from build123d import *

# Parameters (mm, degrees)
F0_R     = 5.35
F1_DEPTH = 1.5
F2_R     = 4.73
F3_DEPTH = 6.16
F4_R     = 1.13
F5_DEPTH = 2.18
F6_R     = 2.97
F7_DEPTH = 13.4
F8_SIZE  = 0.25


with BuildPart() as f1:
    # F0 (on Front) → F1 (new body)
    with BuildSketch(Plane.XZ):
        Circle(F0_R)
    extrude(amount=F1_DEPTH)

    # F2 (on face) → F3 (join)
    with BuildSketch(Plane.XZ.offset(1.5)):
        Circle(F2_R)
    extrude(amount=F3_DEPTH)

    # F4 (on face) → F5 (join)
    with BuildSketch(Plane.XZ.offset(7.66)):
        Circle(F4_R)
    extrude(amount=F5_DEPTH)

    # F6 (on face) → F7 (join)
    with BuildSketch(Plane(origin=(0, 0, 0), x_dir=(-1, 0, 0), z_dir=(0, 1, 0))):
        Circle(F6_R)
    extrude(amount=F7_DEPTH)

    # F8
    f8_edges = [f1.edges().sort_by_distance(p)[0] for p in [
        (-4.73, -7.66, 0),
        (2.97, 13.4, 0),
    ]]
    chamfer(f8_edges, length=F8_SIZE)


solid = f1.part
Work out the finished part from the listing and answer in its coordinate system (mm). A direction names the side the tool comes from. Give positions to 0.01 mm unless a question says otherwise; leave off trailing zeros. Order: outer loops, then holes, each group sorted by start corner. A loop starts at its lowest first (then second) coordinate and runs counter-clockwise, first axis right, second up. Notation, with made-up numbers: M -16.5,75.25 L 30.5,75.25 A24 ccw 30.5,96.25 Z; hole C 15,-38.75 d4. An arc over 180 degrees is marked long. Return JSON: item names as keys, results as strings.
Q1. Which of the six approach directions +Z, -Z, +X, -X, +Y, -Y give full straight-line access (tool end or side, diameter ignored) to faces 1 (the face through (2.3, 0, -2.3)), 2 (the face through (1, -7.66, -1)), 3 (the face through (0, -9.84, 0))?
Answer below:
{"face 1": "+Y", "face 2": "-Y", "face 3": "+Z, -Z, +X, -X, -Y"}
Q2. Find the intervals of material crossed by line 1 along Y through (x, z) = (4, -1.5); line 2 along Y through (x, z) = (0.5, 1.5); line 3 along X through (y, z) = (4.5, -0.75), in increasing order. Write a range as [from, to].
Answer below:
{"line 1": "y = [-7.66, 0]", "line 2": "y = [-7.66, 13.4]", "line 3": "x = [-2.87, 2.87]"}
Q3. Find section C-C, the plane y = -1.25. Write down the section's boundary in (x, z), and give its area (3 significant figures).
Answer below:
{"outline": "C 0,0 d10.7", "area": "89.9 mm^2"}
Q4. Each of these flat-tipped pins is pushed along its axis until it touches: pin 1 (3 mm diameter, centred on x = -2, y = -3.5, fed in from -Z); pin 2 (4 mm diameter, centred on y = -7, z = -2, fed in from +X); pin 3 (2 mm diameter, centred on y = 10, z = 3.5, fed in from -X). Where does it stop, or does it pass through?
Answer below:
{"pin 1": "stops at z = -4.7", "pin 2": "stops at x = 4.73", "pin 3": "stops at x = -1.6"}
Q5. Find section D-D, the plane y = -5.25. Write down the section's boundary in (x, z).
Answer below:
{"outline": "C 0,0 d9.46"}
Q6. Find section B-B, the plane x = 0. Write down the section's boundary in (y, z), and give its area (3 significant figures).
Answer below:
{"outline": "M -9.84,-1.13 L -7.66,-1.13 L -7.66,-4.48 L -7.41,-4.73 L -1.5,-4.73 L -1.5,-5.35 L 0,-5.35 L 0,-2.97 L 13.15,-2.97 L 13.4,-2.72 L 13.4,2.72 L 13.15,2.97 L 0,2.97 L 0,5.35 L -1.5,5.35 L -1.5,4.73 L -7.41,4.73 L -7.66,4.48 L -7.66,1.13 L -9.84,1.13 Z", "area": "159 mm^2"}
Q7. Find section A-A, the plane z = 0. Write down the section's boundary in (x, y).
Answer below:
{"outline": "M -5.35,-1.5 L -4.73,-1.5 L -4.73,-7.41 L -4.48,-7.66 L -1.13,-7.66 L -1.13,-9.84 L 1.13,-9.84 L 1.13,-7.66 L 4.48,-7.66 L 4.73,-7.41 L 4.73,-1.5 L 5.35,-1.5 L 5.35,0 L 2.97,0 L 2.97,13.15 L 2.72,13.4 L -2.72,13.4 L -2.97,13.15 L -2.97,0 L -5.35,0 Z"}
